from build123d import *

# Parameters (mm, degrees)
BOSS_EXTRUDE1_DEPTH = 7.5
SKETCH3_R           = 2.1
CUT_EXTRUDE1_DEPTH  = 5
CIRPATTERN1_COUNT   = 2
CIRPATTERN1_ANGLE   = 90


with BuildPart() as part:
    # Sketch1 → Boss-Extrude1 (new body)
    with BuildSketch(Plane.XY):
        Polygon((12.5, 75), (20, 75), (20, 60), (3.75, 60), (3.75, 0), (-3.75, 0), (-3.75, 60), (-20, 60), (-20, 75), (-12.5, 75), (-12.5, 67.5), (0, 67.5), (12.5, 67.5), align=None)
    extrude(amount=BOSS_EXTRUDE1_DEPTH)

    # Sketch3 → Cut-Extrude1 (cut)
    with BuildSketch(Plane(origin=(0, 75, 0), x_dir=(1, 0, 0), z_dir=(0, 1, 0))):
        with Locations(Location((-16.25, -3.75, 0), (0, 0, 270))):
            Circle(SKETCH3_R)
        with Locations(Location((16.25, -3.75, 0), (0, 0, 270))):
            Circle(SKETCH3_R)
    extrude(amount=-CUT_EXTRUDE1_DEPTH, mode=Mode.SUBTRACT)


with BuildPart() as cirpattern1_1:
    # CirPattern1: pattern copy
    add(part.part.rotate(Axis((0, 0, 3.75), (0, -1, 0)), 1 * CIRPATTERN1_ANGLE / (CIRPATTERN1_COUNT - 1)))


with BuildPart() as part_1:
    add(part.part)

    # Combine1: union CirPattern1_1
    add(cirpattern1_1.part)


solid = part_1.part
Here's how the part is built. I have some questions about the finished solid (model axes, mm). A direction names the side the tool comes from. Give positions to 0.01 mm unless a question says otherwise; leave off trailing zeros. Order: outer loops, then holes, each group sorted by start corner. A loop starts at its lowest first (then second) coordinate and runs counter-clockwise, first axis right, second up. Notation, with made-up numbers: (72.5, 68) -> (86.5, 68) arc R7 ccw to (86.5, 77) -> close; hole circle Ø9 at (1, 78). An arc over 180 degrees is marked (long way). Use a Markdown table: item, result. Add a question column.
Item 1: If we mould it in two halves opening along X, with no side actions, what happens to faces 1 (the face through (12.5, 71, 4)), 2 (the face through (3.75, 66, -10)), 3 (the face through (16, 70, 4)), 4 (the face through (18, 75, 2))? For each: pulls with the +X half, pulls with the -X half, needs draft (parallel to the pull), parting line crosses it, or undercut.
Item 2: Imagine slicing it at D-D on z = 20. Please give me the cut outline in (x, y), plus the area to 3 significant figures.
Item 3: Imagine slicing it at A-A on z = 3.75. Please give me the cut outline in (x, y).
Item 4: Imagine slicing it at C-C on x = 0. Please give me the cut outline in (y, z), plus the area to 4 significant figures.
Item 5: For faces 5 (the face through (-14.48, 72.54, 4.88)), 6 (the face through (0, 30, 0)), 7 (the face through (3.75, 30, 4)), 8 (the face through (-3.75, 66, 18)), which set-ups out of +Z, -Z, +X, -X, +Y, -Y let a thin tool reach every point of the face, with its end or its side?
Item 6: Imagine slicing it at B-B on y = 64. Please give me the cut outline in (x, z).
Item 7: I need wall thicknesses on line 1 (Z direction, x = 0, y = 72.8); line 2 (X direction, y = 73.25, z = 3.75); line 3 (X direction, y = 69.5, z = 3). Which ranges of each line are inside material? Lowest first, please.
Item 8: Will these pins go through, and if not, where does the flat tip stop? pin 1 (4 mm diameter, centred on x = 13.5, z = 4, fed in from -Y); pin 2 (10 mm diameter, centred on x = -10.5, z = -2.5, fed in from +Y); pin 3 (2 mm diameter, centred on x = -1.5, y = 19.5, fed in from -Z); pin 4 (7.5 mm diameter, centred on y = 66.5, z = 13.5, fed in from +X).
Data:
| question | item | result |
|---|---|---|
| 1 | face 1 | undercut |
| 1 | face 2 | pulls with the +X half |
| 1 | face 3 | undercut |
| 1 | face 4 | needs draft |
| 2 | outline | (-3.75, 60) -> (3.75, 60) -> (3.75, 75) -> (2.1, 75) -> (2.1, 70) -> (-2.1, 70) -> (-2.1, 75) -> (-3.75, 75) -> close |
| 2 | area | 91.5 mm² |
| 3 | outline | (-20, 60) -> (-3.75, 60) -> (-3.75, 0) -> (3.75, 0) -> (3.75, 60) -> (20, 60) -> (20, 75) -> (18.35, 75) -> (18.35, 70) -> (14.15, 70) -> (14.15, 75) -> (12.5, 75) -> (12.5, 67.5) -> (-12.5, 67.5) -> (-12.5, 75) -> (-14.15, 75) -> (-14.15, 70) -> (-18.35, 70) -> (-18.35, 75) -> (-20, 75) -> close |
| 4 | outline | (0, 0) -> (60, 0) -> (60, -16.25) -> (75, -16.25) -> (75, -14.6) -> (70, -14.6) -> (70, -10.4) -> (75, -10.4) -> (75, -8.75) -> (67.5, -8.75) -> (67.5, 16.25) -> (75, 16.25) -> (75, 17.9) -> (70, 17.9) -> (70, 22.1) -> (75, 22.1) -> (75, 23.75) -> (60, 23.75) -> (60, 7.5) -> (0, 7.5) -> close |
| 4 | area | 820.5 mm² |
| 5 | face 5 | +Y |
| 5 | face 6 | -Z, +X, -X, -Y |
| 5 | face 7 | +Z, -Z, +X, -Y |
| 5 | face 8 | +Z, -X, +Y, -Y |
| 6 | outline | (-20, 0) -> (-3.75, 0) -> (-3.75, -16.25) -> (3.75, -16.25) -> (3.75, 0) -> (20, 0) -> (20, 7.5) -> (3.75, 7.5) -> (3.75, 23.75) -> (-3.75, 23.75) -> (-3.75, 7.5) -> (-20, 7.5) -> close |
| 7 | line 1 | z = -16.25 to -14.6, -10.4 to -8.75, 16.25 to 17.9, 22.1 to 23.75 |
| 7 | line 2 | x = -20 to -18.35, -14.15 to -12.5, 12.5 to 14.15, 18.35 to 20 |
| 7 | line 3 | x = -20 to -12.5, 12.5 to 20 |
| 8 | pin 1 | stops at y = 60 |
| 8 | pin 2 | stops at y = 75 |
| 8 | pin 3 | stops at z = 0 |
| 8 | pin 4 | stops at x = 3.75 |
